Can you work these out from the model? Positions are in its coordinate system, mm. Face numbers are marked on the shaded views. A direction names the side the tool comes from. Round coordinates to 2 decimals unless told otherwise and drop trailing zeros. Write each loop counter-clockwise with the first axis right and the second up, starting at its lowest first coordinate (ties: lowest second). Pieces come first, ordered by that corner, then holes. Notation, with made-up numbers: M 57.5,33 L 86.5,33 A30 ccw 86.5,56 Z; hole C 7.25,-4 d1. An arc over 180 degrees is marked long. Use one line per item in the form item = value. Start each with the question number.
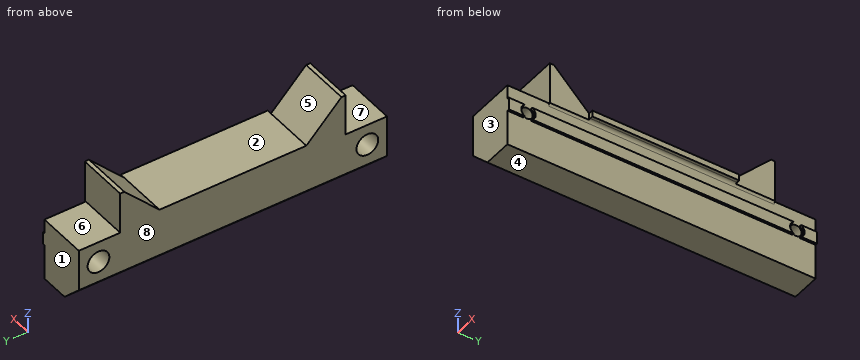
```python
from build123d import *
from build123d.topology import SkipClean

# Parameters (mm, degrees)
BOSS_EXTRUDE1_DEPTH            = 7.2
SKETCH2_R                      = 1.1
CUT_EXTRUDE1_DEPTH             = 99.880748885
SKETCH3_R                      = 2.25
CUT_EXTRUDE2_DEPTH             = 5.5
BOSS_EXTRUDE2_DEPTH            = 3
FILLET1_R                      = 11
BOSS_EXTRUDE3_DEPTH            = 43
BOSS_EXTRUDE4_DEPTH            = 30
FILLET2_R                      = 1.5
SKETCH7_R                      = 2.75
CUT_EXTRUDE3_DEPTH             = 179.693144804
SKETCH8_R                      = 5.25
CUT_EXTRUDE4_DEPTH             = 5
CUT_EXTRUDE6_START             = -2.5
SKETCH10_R                     = 5.25
CUT_EXTRUDE6_DEPTH             = 2.5
CHAMFER1_SIZE                  = 2.5
CUT_EXTRUDE5_REACH             = 170.548
SKETCH9_R                      = 3.5
CUT_EXTRUDE5_DIRECTION_2_REACH = 170.548
CUT_EXTRUDE7_DEPTH             = 105.056727317
CUT_EXTRUDE8_DEPTH             = 20
BOSS_EXTRUDE6_DEPTH            = 17
SKETCH15_R                     = 5.25
BOSS_EXTRUDE7_DEPTH            = 10
CHAMFER3_SIZE                  = 10
BOSS_EXTRUDE5_DEPTH            = 17.55
SKETCH16_W                     = 1.5
SKETCH16_H                     = 19
CUT_EXTRUDE9_DEPTH             = 2.3
BOSS_EXTRUDE8_DEPTH            = 4
BOSS_EXTRUDE9_DEPTH            = 31.5


with BuildPart() as part:
    # Sketch1 → Boss-Extrude1 (new body)
    with BuildSketch(Plane.XY):
        Polygon((74.75, 0), (-74.75, 0), (-74.75, 30), (-88.75, 30), (-88.75, -13), (84.25, -13), (84.25, 17), (74.75, 17), align=None)
    extrude(amount=BOSS_EXTRUDE1_DEPTH)

    # Sketch2 → Cut-Extrude1 (cut, through all)
    with BuildSketch(Plane.XZ.offset(13)):
        with Locations(Location((-56.25, 4.5, 0), (0, 0, 270))):
            Circle(SKETCH2_R)
        with Locations(Location((37.75, 4.5, 0), (0, 0, 270))):
            Circle(SKETCH2_R)
    extrude(amount=-CUT_EXTRUDE1_DEPTH, mode=Mode.SUBTRACT)

    # Sketch3 → Cut-Extrude2 (cut)
    with BuildSketch(Plane.XZ.offset(13)):
        with Locations(Location((-56.25, 4.5, 0), (0, 0, 270))):
            Circle(SKETCH3_R)
        with Locations(Location((37.75, 4.5, 0), (0, 0, 270))):
            Circle(SKETCH3_R)
    extrude(amount=-CUT_EXTRUDE2_DEPTH, mode=Mode.SUBTRACT)

    # Sketch4 → Boss-Extrude2 (add)
    with BuildSketch(Plane.XY.offset(7.2)):
        Polygon((-88.75, -13), (84.25, -13), (84.25, 2.989373151), (84.25, 17), (74.75, 17), (74.75, 6), (-74.75, 6), (-74.75, 30), (-88.75, 30), align=None)
    extrude(amount=BOSS_EXTRUDE2_DEPTH)

    # Fillet1
    fillet1_edges = [part.edges().sort_by_distance(p)[0] for p in [
        (74.75, 6, 8.7),
        (-74.75, 6, 8.7),
    ]]
    fillet(fillet1_edges, radius=FILLET1_R - 0.0001)  # a hair under: the kernel refuses the full size

    # Sketch5 → Boss-Extrude3 (add)
    with BuildSketch(Plane.XZ.offset(13)):
        Polygon((-74.75, 30.2), (-71.75, 30.2), (-71.75, 33.2), (-88.75, 33.2), (-88.75, 10.2), (-74.75, 10.2), (-74.75, 17.2), (-73.75, 17.2), (-73.75, 23.2), (-74.75, 23.2), align=None)
    extrude(amount=-BOSS_EXTRUDE3_DEPTH)

    # Sketch6 → Boss-Extrude4 (add)
    with BuildSketch(Plane.XZ.offset(13)):
        Polygon((74.75, 10.2), (74.75, 17.2), (73.75, 17.2), (73.75, 23.2), (74.75, 23.2), (74.75, 30.2), (71.75, 30.2), (71.75, 33.2), (84.25, 33.2), (84.25, 10.2), align=None)
    extrude(amount=-BOSS_EXTRUDE4_DEPTH)

    # Fillet2
    fillet2_edges = [part.edges().sort_by_distance(p)[0] for p in [
        (74.75, 1.99995, 10.2),
        (74.75, 2, 30.2),
        (-74.75, 1.99995, 10.2),
        (-74.75, 8.5, 30.2),
    ]]
    fillet(fillet2_edges, radius=FILLET2_R)

    # Sketch7 → Cut-Extrude3 (cut, through all)
    with BuildSketch(Plane(origin=(84.25, 0, 0), x_dir=(0, 0, -1), z_dir=(1, 0, 0))):
        with Locations((-20.2, -3.5)):
            Circle(SKETCH7_R)
    extrude(amount=-CUT_EXTRUDE3_DEPTH, mode=Mode.SUBTRACT)

    # Sketch8 → Cut-Extrude4 (cut)
    with BuildSketch(Plane(origin=(84.25, 0, 0), x_dir=(0, 0, -1), z_dir=(1, 0, 0))):
        with Locations((-20.2, -3.5)):
            Circle(SKETCH8_R)
    extrude(amount=-CUT_EXTRUDE4_DEPTH, mode=Mode.SUBTRACT)

    # Sketch10 → Cut-Extrude6 (cut)
    with BuildSketch(Plane.ZY.offset(88.75).offset(CUT_EXTRUDE6_START)):
        with Locations(Location((20.2, -3.5, 0), (0, 0, 180))):
            Circle(SKETCH10_R)
    extrude(amount=CUT_EXTRUDE6_DEPTH, mode=Mode.SUBTRACT)

    # Chamfer1
    chamfer1_edges = [part.edges().sort_by_distance(p)[0] for p in [
        (79.25, -3.5, 22.95),
        (-86.25, -3.5, 22.95),
    ]]
    chamfer(chamfer1_edges, length=CHAMFER1_SIZE - 0.0001)  # a hair under: the kernel refuses the full size

    # Cut-Extrude5: up to this face of the body (flat: up to its plane)
    cut_extrude5_end = Plane(part.part.faces().sort_by_distance((74.75, 2, 25.95))[0])
    # Sketch9 → Cut-Extrude5 (cut, up to the picked face)
    with BuildSketch(Plane.ZY.offset(-73.75), mode=Mode.PRIVATE) as cut_extrude5_sk1:
        with Locations((20.2, -3.5)):
            Circle(SKETCH9_R)
    cut_extrude5_tool1 = split(extrude(cut_extrude5_sk1.sketch, amount=-CUT_EXTRUDE5_REACH, mode=Mode.PRIVATE), bisect_by=cut_extrude5_end, keep=Keep.BOTH, mode=Mode.PRIVATE)
    add(cut_extrude5_tool1.solids().sort_by(Axis((73.75, -3.5, 20.2), (1, 0, 0)))[0], mode=Mode.SUBTRACT)

    # Cut-Extrude5 direction 2: up to this face of the body (flat: up to its plane)
    cut_extrude5_direction_2_end = Plane(part.part.faces().sort_by_distance((-74.75, 8.5, 25.95))[0])
    # Sketch9 → Cut-Extrude5 direction 2 (cut, up to the picked face)
    with BuildSketch(Plane.ZY.offset(-73.75), mode=Mode.PRIVATE) as cut_extrude5_direction_2_sk1:
        with Locations((20.2, -3.5)):
            Circle(SKETCH9_R)
    cut_extrude5_direction_2_tool1 = split(extrude(cut_extrude5_direction_2_sk1.sketch, amount=CUT_EXTRUDE5_DIRECTION_2_REACH, mode=Mode.PRIVATE), bisect_by=cut_extrude5_direction_2_end, keep=Keep.BOTH, mode=Mode.PRIVATE)
    add(cut_extrude5_direction_2_tool1.solids().sort_by(Axis((73.75, -3.5, 20.2), (-1, 0, 0)))[0], mode=Mode.SUBTRACT)


with BuildPart() as body_2:
    # Mirror1: mirrored copy
    add(part.part.mirror(Plane(origin=(-88.75, -13, 7.2), x_dir=(0, 0, 1), z_dir=(0, 1, 0))))

    # Sketch11 → Cut-Extrude7 (cut, through all)
    with BuildSketch(Plane(origin=(0, -13, 0), x_dir=(1, 0, 0), z_dir=(0, 1, 0))):
        Polygon((71.75, -33.2), (71.75, -17.2), (-74.75, -17.2), (-74.75, 0), (71.75, 0), (84.25, 0), (84.25, -33.2), align=None)
    extrude(amount=-CUT_EXTRUDE7_DEPTH, mode=Mode.SUBTRACT)

    # Sketch13 → Cut-Extrude8 (cut)
    with BuildSketch(Plane(origin=(0, -13, 0), x_dir=(1, 0, 0), z_dir=(0, 1, 0))):
        Polygon((-88.75, -30.2), (-74.75, -30.2), (-74.75, -28.7), (-71.75, -28.7), (-71.75, -30.2), (-71.75, -33.2), (-88.75, -33.2), align=None)
    extrude(amount=-CUT_EXTRUDE8_DEPTH, mode=Mode.SUBTRACT)

    # Sketch14 → Boss-Extrude6 (add)
    with BuildSketch(Plane.ZY.offset(88.75)):
        Polygon((33.2, -33), (50.2, -33), (50.2, -35), (35.2, -50), (33.2, -52), (33.2, -50), align=None)
    extrude(amount=-BOSS_EXTRUDE6_DEPTH)

    # Sketch15 → Boss-Extrude7 (add)
    with SkipClean():  # the faces are left unmerged after this step: merging them gives an invalid solid
        with BuildSketch(Plane.ZY.offset(88.75)):
            Polygon((33.2, -52), (0, -52), (0, -13), (30.2, -13), (30.2, -33), (50.2, -33), (50.2, -35), align=None)
            with Locations((20.2, -22.5)):
                Circle(SKETCH15_R, mode=Mode.SUBTRACT)
        extrude(amount=BOSS_EXTRUDE7_DEPTH)
    add(body_2.part.scale(1), mode=Mode.REPLACE)  # the faces are merged on a copy

    # Chamfer3
    chamfer3_edges = [body_2.edges().sort_by_distance(p)[0] for p in [
        (-98.75, -32.5, 0),
    ]]
    chamfer(chamfer3_edges, length=CHAMFER3_SIZE)

    # Sketch12 → Boss-Extrude5 (add)
    with SkipClean():  # the faces are left unmerged after this step: merging them gives an invalid solid
        with BuildSketch(Plane.XZ.offset(56)):
            with BuildLine():
                Line((-88.75, 0), (-74.75, 0))
                Line((-74.75, 0), (-74.75, 17.2))
                Line((-74.75, 17.2), (-73.75, 17.2))
                Line((-73.75, 17.2), (-73.75, 23.2))
                Line((-73.75, 23.2), (-74.75, 23.2))
                Line((-74.75, 23.2), (-74.75, 28.7))
                ThreePointArc((-74.75, 28.7), (-74.310660172, 29.760660172), (-73.25, 30.2))
                Line((-73.25, 30.2), (-71.75, 30.2))
                Line((-71.75, 30.2), (-71.75, 33.2))
                Line((-71.75, 33.2), (-88.75, 33.2))
                Line((-88.75, 33.2), (-88.75, 0))
            make_face()
        extrude(amount=-BOSS_EXTRUDE5_DEPTH)

    # Sketch16 → Cut-Extrude9 (cut)
    with SkipClean():  # the faces are left unmerged after this step: merging them gives an invalid solid
        with BuildSketch(Plane(origin=(-71.75, 0, 0), x_dir=(0, 0, -1), z_dir=(1, 0, 0))):
            Polygon((-33.2, -52), (-30.2, -52), (-30.2, -33), (-50.2, -33), (-50.2, -35), align=None)
            with Locations((-29.45, -42.5)):
                Rectangle(SKETCH16_W, SKETCH16_H)
        extrude(amount=-CUT_EXTRUDE9_DEPTH, mode=Mode.SUBTRACT)

    # Sketch18 → Boss-Extrude8 (add)
    with SkipClean():  # the faces are left unmerged after this step: merging them gives an invalid solid
        with BuildSketch(Plane.XZ.offset(52)):
            Polygon((-98.75, 33.2), (-98.75, 10), (-88.75, 0), (-88.75, 33.2), align=None)
        extrude(amount=BOSS_EXTRUDE8_DEPTH)

    # Sketch19 → Boss-Extrude9 (add)
    with SkipClean():  # the faces are left unmerged after this step: merging them gives an invalid solid
        with BuildSketch(Plane.XZ.offset(56)):
            with BuildLine():
                Line((-88.75, 0), (-74.75, 0))
                Line((-74.75, 0), (-74.75, 17.2))
                Line((-74.75, 17.2), (-73.75, 17.2))
                Line((-73.75, 17.2), (-73.75, 23.2))
                Line((-73.75, 23.2), (-74.75, 23.2))
                Line((-74.75, 23.2), (-74.75, 28.7))
                ThreePointArc((-74.75, 28.7), (-74.310660172, 29.760660172), (-73.25, 30.2))
                Line((-73.25, 30.2), (-71.75, 30.2))
                Line((-71.75, 30.2), (-71.75, 33.2))
                Line((-71.75, 33.2), (-98.75, 33.2))
                Line((-98.75, 33.2), (-98.75, 10))
                Line((-98.75, 10), (-88.75, 0))
            make_face()
        extrude(amount=BOSS_EXTRUDE9_DEPTH)

    # Mirror2: body 2 across plane


with BuildPart() as body_2_1:
    with SkipClean():  # the faces are left unmerged after this step: merging them gives an invalid solid
        add(body_2.part)
        add(body_2.part.mirror(Plane.ZX.offset(-87.5)))


solid = body_2_1.part
```
1. If we section it at A-A (x = -79.75): List the corners of the cut face in (y, z) for me.
2. Please list where these lines run through material, in increasing order: line 1 along Y through (x, z) = (-92.25, 20.2); line 2 along Z through (x, y) = (-88.2, -152.5); line 3 along Z through (x, y) = (-80.5, -22.5).
3. Which directions (+Z, -Z, +X, -X, +Y, -Y) give clear straight access to the entire face, cutting with the end or side of a thin tool? Please do the marked faces 4, 5, 6, 7 and 8.
4. If we section it at B-B (z = 20.2): State how many separate pieces and enclosed holes the cut face has, and give its area (3 significant figures).
5. If we mould it in two halves opening along Y, with no side actions, what happens to the marked faces 1, 2 and 3? For each: pulls with the +Y half, pulls with the -Y half, needs draft (parallel to the pull), parting line crosses it, or undercut.
6. If we section it at D-D (z = 45.5): List the corners of the cut face in (x, y) for me, and give its area (3 significant figures).
7. Will these pins go through, and if not, where does the flat tip stop? pin 1 (8.5 mm diameter, centred on y = -24, z = 18, fed in from -X); pin 2 (0.5 mm diameter, centred on x = -74, y = -157.5, fed in from +Z); pin 3 (6.5 mm diameter, centred on y = -22.5, z = 20.2, fed in from -X); pin 4 (13.5 mm diameter, centred on y = -152.5, z = 20.2, fed in from +X).
Model answer:
q1.outline = M -162,0 L -13,0 L -13,30.2 L -33,30.2 L -33,50.2 L -35,50.2 L -52,33.2 L -123,33.2 L -140,50.2 L -142,50.2 L -142,30.2 L -162,30.2 Z; hole C -152.5,20.2 d5.5; hole C -22.5,20.2 d5.5
q2.line_1 = -162 to -157.75, -147.25 to -27.75, -17.25 to -13
q2.line_2 = 0 to 14.95, 25.45 to 30.2
q2.line_3 = 0 to 17.45, 22.95 to 30.2
q3.face_4 = -Z, +X, -X, +Y, -Y
q3.face_5 = +Z, +X, -X
q3.face_6 = +Z, +X, -X, +Y
q3.face_7 = +Z, +X, -X, -Y
q3.face_8 = +Z, -Z, -X, +Y, -Y
q4.separate_pieces = 3
q4.enclosed_holes = 0
q4.area = 3,310 mm2
q5.face_1 = pulls with the +Y half
q5.face_2 = undercut
q5.face_3 = pulls with the -Y half
q6.outline = M -98.75,-142 L -74.05,-142 L -74.05,-135.3 L -98.75,-135.3 Z; M -98.75,-39.7 L -74.05,-39.7 L -74.05,-33 L -98.75,-33 Z
q6.area = 331 mm2
q7.pin_1 = -98.75
q7.pin_2 = 23.2
q7.pin_3 = -84.25
q7.pin_4 = -73.75
